Part model, mm, in its own coordinate system. A direction names the side the tool comes from. Give positions to 0.01 mm unless a question says otherwise; leave off trailing zeros. Order: outer loops, then holes, each group sorted by start corner. A loop starts at its lowest first (then second) coordinate and runs counter-clockwise, first axis right, second up. Notation, with made-up numbers: (62.5, 16) -> (92.5, 16) arc R18 ccw to (92.5, 44) -> close; hole circle Ø3 at (36, -11.75). An arc over 180 degrees is marked (long way). Write item = value, one per line. Start each with the question number.
Item 1: Drill centre lines: line 1 along X through (y, z) = (22, 29.5); line 2 along Y through (x, z) = (27, 34.5); line 3 along Z through (x, y) = (-20.5, 49). Where is each one in solid material? Low to high.
Item 2: Tool access for faces 1 (the face through (-35.5, 12, 34)), 2 (the face through (11, 48, 37)), 3 (the face through (90.5, 27, 26)), 4 (the face through (60.5, 13, 34)), 5 (the face through (12, 50.5, 34)): list every direction of +Z, -Z, +X, -X, +Y, -Y with a clear straight run to the whole face (end or side of a thin tool).
Item 3: Band-saw the part on A-A on y = 8.5. Count the separate pieces of the cut face and the enclosed holes in it, plus the area to 3 significant figures.
Item 4: Flat gauge pins, fed straight in: P1, Ø4, axis at x = -22.5, y = 20.5, coming from the +Z side; P2, Ø0.6, axis at x = -31.5, y = 21.5, coming from the +Z side; P3, Ø1, axis at x = 56.5, y = -0.5, coming from the +Z side. Where does each tip first touch, or does it go through?
Item 5: Band-saw the part on B-B on y = 71. Write the cut outline in (x, z).
Autodesk Fusion 360 part; units mm, degrees
sketch "Bottom opening" plane through (0, 0, 0) normal (0, 0, 1) x (1, 0, 0)
  line L0 (0, 0) -> (25, 0)
  line L1 (25, 0) -> (25, 25)
  line L2 (25, 25) -> (0, 25)
  line L3 (0, 25) -> (0, 0)
  line L4 (-4, 29) -> (29, 29)
  line L5 (29, 29) -> (29, -4)
  line L6 (29, -4) -> (-4, -4)
  line L7 (-4, -4) -> (-4, 29)
  dimension "d3" = 25
  dimension "d4" = 25
  dimension "d5" = 4
  dimension "d6" = 4
  dimension "d7" = 4
  dimension "d8" = 4
ref_plane "WorkPlane1" through (0, 0, 37) normal (0, 0, 1) x (1, 0, 0)
sketch "Top opening" plane through (0, 0, 37) normal (0, 0, 1) x (1, 0, 0)
  line L0 (25, 25) -> (0, 25)
  line L1 (25, 0) -> (25, 25)
  line L2 (0, 0) -> (25, 0)
  line L3 (0, 25) -> (0, 0)
  line L4 (-4, 29) -> (29, 29)
  line L5 (29, -4) -> (-4, -4)
  line L6 (29, 29) -> (29, -4)
  line L7 (-4, -4) -> (-4, 29)
  line L8 (-32.5, 47.5) -> (57.5, 47.5)
  line L9 (57.5, 47.5) -> (57.5, -22.5)
  line L10 (57.5, -22.5) -> (-32.5, -22.5)
  line L11 (-32.5, -22.5) -> (-32.5, 47.5)
  line L12 (-35.5, 50.5) -> (60.5, 50.5)
  line L13 (60.5, 50.5) -> (60.5, -25.5)
  line L14 (60.5, -25.5) -> (-35.5, -25.5)
  line L15 (-35.5, -25.5) -> (-35.5, 50.5)
  line L16 (-36.5, 51.5) -> (61.5, 51.5)
  line L17 (61.5, 51.5) -> (61.5, -26.5)
  line L18 (61.5, -26.5) -> (-36.5, -26.5)
  line L19 (-36.5, -26.5) -> (-36.5, 51.5)
  dimension "d14" = 3
  dimension "d15" = 4
  dimension "d16" = 3
  dimension "d17" = 4
  dimension "d18" = 90
  dimension "d19" = 70
  dimension "d20" = 3
  dimension "d21" = 4
  dimension "d22" = 3
  dimension "d23" = 4
  dimension "d24" = 28.5
  dimension "d25" = 28.5
  dimension "d26" = 18.5
  dimension "d27" = 18.5
loft "Loft1" add profiles "Top opening", "Bottom opening" section 1 contours L8 L9 L10 L11 | L12 L13 L14 L15 | L16 L17 L18 L19 section 2 contours L0 L1 L2 L3 | L4 L5 L6 L7
extrude "Extrude1" cut sketch "Top opening" against normal blind 6 contours L16 L17 L18 L19
sketch "Support lip" plane through (60.5, 0, 0) normal (1, 0, 0) x (0, 1, 0)
  line L0 (-25.5, 35.8615) -> (50.5, 35.8615)
  line L1 (50.5, 35.8615) -> (50.5, 37)
  line L2 (50.5, 37) -> (-25.5, 37)
  line L3 (-25.5, 37) -> (-25.5, 35.8615)
  line L4 (-25.5, 31) -> (80.5, 31)
  line L5 (80.5, 31) -> (80.5, 21)
  line L6 (80.5, 21) -> (-25.5, 21)
  line L7 (-25.5, 21) -> (-25.5, 31)
  dimension "d31" = 6
  dimension "d34" = 10
  dimension "d35" = 30
extrude "Extrude2" add sketch "Support lip" along normal blind 30 and the other way blind 126 contours L4 L5 L6 L7
loft "Loft2" cut profiles "Top opening", "Bottom opening" section 1 contours L8 L9 L10 L11 section 2 contours L0 L1 L2 L3
extrude "Extrude3" add 1 faces at (-2.5, 49.5, 37) along direction (0, 0, -1) blind 6
equation "bottom_outlet_size = 25 mm"
equation "hopper_wall_thickness = 4 mm"
equation "d3 = bottom_outlet_size"
equation "d4 = bottom_outlet_size"
equation "d5 = hopper_wall_thickness"
equation "d6 = hopper_wall_thickness"
equation "d7 = hopper_wall_thickness"
equation "d8 = hopper_wall_thickness"
equation "hopper_height = 37 mm"
equation "d10 = hopper_height"
equation "acrylic_thickness = 3 mm"
equation "top_outlet_width = 90 mm"
equation "top_outlet_depth = 70 mm"
equation "d14 = acrylic_thickness"
equation "d15 = hopper_wall_thickness"
equation "d16 = acrylic_thickness"
equation "d17 = hopper_wall_thickness"
equation "d18 = top_outlet_width"
equation "d19 = top_outlet_depth"
equation "d20 = acrylic_thickness"
equation "d21 = hopper_wall_thickness"
equation "d22 = acrylic_thickness"
equation "d23 = hopper_wall_thickness"
equation "d24 = ( top_outlet_width - ( bottom_outlet_size + 2 * hopper_wall_thickness ) ) / 2"
equation "d26 = ( top_outlet_depth - ( bottom_outlet_size + 2 * hopper_wall_thickness ) ) / 2"
equation "MDF_thickness = 6 mm"
equation "d31 = MDF_thickness"
equation "support_lip_width = 30 mm"
equation "support_lip_thickness = 10 mm"
equation "d34 = support_lip_thickness"
equation "d35 = support_lip_width"
equation "d36 = support_lip_width"
equation "d38 = ( top_outlet_width + 2 * acrylic_thickness ) + support_lip_width"
Values found:
q1.line_1 = -65.5 to -25.91, 50.91 to 90.5
q1.line_2 = -25.5 to -20.98, 45.98 to 50.5
q1.line_3 = 21 to 37
q2.face_1 = +Z, -X, +Y, -Y
q2.face_2 = +Z, +X, -X, +Y, -Y
q2.face_3 = +Z, -Z, +X, +Y, -Y
q2.face_4 = +Z, +X, +Y, -Y
q2.face_5 = +Z, +X, -X, +Y
q3.separate_pieces = 2
q3.enclosed_holes = 2
q3.area = 1,090 mm^2
q4.P1 = 27.89
q4.P2 = 36.2
q4.P3 = 36.43
q5.outline = (-65.5, 21) -> (90.5, 21) -> (90.5, 31) -> (-65.5, 31) -> close
